from build123d import *

# Parameters (mm, degrees)
F0_W     = 1000
F0_H     = 500
F0_W_2   = 350
F0_H_2   = 150
F1_DEPTH = 8
F2_W     = 8
F2_H     = 500
F3_DEPTH = 150
F4_R     = 8
F5_R     = 6.5
F6_DEPTH = 1200


with BuildPart() as f1:
    # F0 (on Top) → F1 (new body)
    with BuildSketch(Plane.XY):
        Rectangle(F0_W, F0_H)
        with Locations((-255, -105)):
            Rectangle(F0_W_2, F0_H_2, mode=Mode.SUBTRACT)
        with Locations((255, -105)):
            Rectangle(F0_W_2, F0_H_2, mode=Mode.SUBTRACT)
        with Locations((-255, 105)):
            Rectangle(F0_W_2, F0_H_2, mode=Mode.SUBTRACT)
        with Locations((255, 105)):
            Rectangle(F0_W_2, F0_H_2, mode=Mode.SUBTRACT)
    extrude(amount=F1_DEPTH)

    # F2 (on face) → F3 (join)
    with BuildSketch(Plane.XY.offset(8)):
        with Locations((-496, 0)):
            Rectangle(F2_W, F2_H)
        with Locations((496, 0)):
            Rectangle(F2_W, F2_H)
    extrude(amount=F3_DEPTH)

    # F4
    f4_edges = [f1.edges().sort_by_distance(p)[0] for p in [
        (-500, 0, 0),
        (500, 0, 0),
    ]]
    fillet(f4_edges, radius=F4_R)

    # F5 (on face) → F6 (cut)
    with BuildSketch(Plane(origin=(-500, 0, 0), x_dir=(0, -1, 0), z_dir=(-1, 0, 0))):
        with Locations((-200, 40)):
            Circle(F5_R)
        with Locations((-200, 118)):
            Circle(F5_R)
        with Locations((200, 118)):
            Circle(F5_R)
        with Locations((200, 40)):
            Circle(F5_R)
    extrude(amount=-F6_DEPTH, mode=Mode.SUBTRACT)


solid = f1.part
The model under review builds one solid part; all positions refer to its coordinate system, in mm. A direction names the side the tool comes from. Round coordinates to 2 decimals unless told otherwise and drop trailing zeros. Loops run counter-clockwise (first coordinate to the right, second up) from the corner with the lowest first, then second, coordinate; pieces in that order, holes last. Notation, with made-up numbers: M 75.5,83.5 L 131.5,83.5 A27 cw 131.5,121.5 Z; hole C 33.25,74.5 d1. An arc over 180 degrees is marked long. Answer as CSV lines item,"result".
1. To check wall thickness, follow L1, parallel to X at y = 28, z = 38.5; L2, parallel to Z at x = -317.5, y = -225. State the ranges of each line that lie inside material, in increasing order. Write a range as [from, to].
Outcome:
L1,"x = [-500, -492], [492, 500]"
L2,"z = [0, 8]"
2. We need section D-D (y = -217). Give the boundary of the cut face in (x, z), plus the area to 3 significant figures.
Outcome:
outline,"M -500,8 A8 ccw -492,0 L 492,0 A8 ccw 500,8 L 500,158 L 492,158 L 492,8 L -492,8 L -492,158 L -500,158 Z"
area,"10,400 mm2"
3. We need section B-B (y = -144). Give the boundary of the cut face in (x, z), plus the area to 3 significant figures.
Outcome:
outline,"M -500,8 A8 ccw -492,0 L -430,0 L -430,8 L -492,8 L -492,158 L -500,158 Z; M -80,0 L 80,0 L 80,8 L -80,8 Z; M 430,0 L 492,0 A8 ccw 500,8 L 500,158 L 492,158 L 492,8 L 430,8 Z"
area,"4,770 mm2"
4. We need section C-C (x = -399). Give the boundary of the cut face in (y, z).
Outcome:
outline,"M -250,0 L -180,0 L -180,8 L -250,8 Z; M -30,0 L 30,0 L 30,8 L -30,8 Z; M 180,0 L 250,0 L 250,8 L 180,8 Z"
5. Insertion check: pin 1 Ø2.5 at (y, z) = (-89, 4.5) entering from -X; pin 2 Ø2.5 at (y, z) = (102.5, 3) entering from +X; pin 3 Ø2 at (x, y) = (3.5, -169) entering from +Z. Each pin has a flat end and moves straight along its axis. Give the tip position at first contact, or say it passes through.
Outcome:
pin 1,"stops at x = -499.68"
pin 2,"stops at x = 499.07"
pin 3,"stops at z = 8"
6. For faces 1 (the face through (492, -3, 82)), 2 (the face through (-2, -250, 3)), list the 3-axis set-ups (+Z, -Z, +X, -X, +Y, -Y) from which the entire face can be reached by the end or side of a thin tool; tool diameter is ignored.
Outcome:
face 1,"+Z, +Y, -Y"
face 2,"+Z, -Z, +X, -X, -Y"
7. We need section A-A (z = 57.5). Give the boundary of the cut face in (x, y).
Outcome:
outline,"M -500,-250 L -492,-250 L -492,250 L -500,250 Z; M 492,-250 L 500,-250 L 500,250 L 492,250 Z"
